```python
from build123d import *

# Parameters (mm, degrees)
F0_R     = 5.624793
F0_R_2   = 8.743876
F0_R_3   = 6.820271
F0_R_4   = 3.661746
F0_R_5   = 5.429622
F0_R_6   = 8.809277
F0_R_7   = 6.306028
F0_R_8   = 3.649185
F0_R_9   = 9.51591
F0_R_10  = 3.388182
F0_R_11  = 3.649186
F0_R_12  = 4.291104
F0_R_13  = 3.488347
F0_R_14  = 4.625832
F0_R_15  = 4.5204
F0_R_16  = 5.057367
F1_DEPTH = 7.62


with BuildPart() as f1:
    # F0 (on Top) → F1 (new body)
    with BuildSketch(Plane.XY):
        with BuildLine():
            ThreePointArc((38.1, 26.47022), (28.9765, 28.732993), (28.190642, 38.1))
            Line((28.190642, 38.1), (16.499434, 38.1))
            ThreePointArc((16.499434, 38.1), (16.874, 36.915099), (17.000607, 35.678871))
            ThreePointArc((17.000607, 35.678871), (9.665649, 29.706748), (5.304319, 38.1))
            Line((5.304319, 38.1), (-38.1, 38.1))
            Line((-38.1, 38.1), (-38.1, 17.180183))
            ThreePointArc((-38.1, 17.180183), (-32.694602, 14.941194), (-30.455614, 9.535796))
            ThreePointArc((-30.455614, 9.535796), (-32.694602, 4.130398), (-38.1, 1.89141))
            Line((-38.1, 1.89141), (-38.1, -13.310762))
            ThreePointArc((-38.1, -13.310762), (-34.005794, -13.280793), (-31.949991, -16.821569))
            ThreePointArc((-31.949991, -16.821569), (-34.005794, -20.362345), (-38.1, -20.332376))
            Line((-38.1, -20.332376), (-38.1, -26.536592))
            ThreePointArc((-38.1, -26.536592), (-28.827146, -26.010312), (-24.032091, -33.964571))
            ThreePointArc((-24.032091, -33.964571), (-24.287465, -36.092705), (-25.039087, -38.1))
            Line((-25.039087, -38.1), (-6.594518, -38.1))
            ThreePointArc((-6.594518, -38.1), (-5.905659, -25.985243), (4.486227, -32.25027))
            ThreePointArc((4.486227, -32.25027), (3.666791, -35.557694), (1.398047, -38.1))
            Line((1.398047, -38.1), (38.1, -38.1))
            Line((38.1, -38.1), (38.1, -34.461013))
            ThreePointArc((38.1, -34.461013), (22.042395, -27.750231), (38.1, -21.039449))
            Line((38.1, -21.039449), (38.1, 7.983235))
            ThreePointArc((38.1, 7.983235), (29.755205, 13.178684), (38.1, 18.374132))
            Line((38.1, 18.374132), (38.1, 26.47022))
        make_face()
        with Locations((-27.455587, -5.678618)):
            Circle(F0_R, mode=Mode.SUBTRACT)
        with Locations((-17.169787, -20.250168)):
            Circle(F0_R_2, mode=Mode.SUBTRACT)
        with Locations((-11.598311, -3.535743)):
            Circle(F0_R_3, mode=Mode.SUBTRACT)
        with Locations((10.044727, -23.035906)):
            Circle(F0_R_4, mode=Mode.SUBTRACT)
        with Locations((0, -18.321581)):
            Circle(F0_R_5, mode=Mode.SUBTRACT)
        with Locations((8.544715, -1.607155)):
            Circle(F0_R_6, mode=Mode.SUBTRACT)
        with Locations((24.401991, -10.392943)):
            Circle(F0_R_7, mode=Mode.SUBTRACT)
        with Locations((-4.312536, 6.750058)):
            Circle(F0_R_8, mode=Mode.SUBTRACT)
        with Locations((-19.526949, 19.178735)):
            Circle(F0_R_9, mode=Mode.SUBTRACT)
        with Locations((-32.812774, 31.607412)):
            Circle(F0_R_10, mode=Mode.SUBTRACT)
        with Locations((-2.598236, 26.893085)):
            Circle(F0_R_11, mode=Mode.SUBTRACT)
        with Locations((-13.741186, 33.107422)):
            Circle(F0_R_12, mode=Mode.SUBTRACT)
        with Locations((11.759028, 12.535821)):
            Circle(F0_R_13, mode=Mode.SUBTRACT)
        with Locations((24.616279, 8.464358)):
            Circle(F0_R_14, mode=Mode.SUBTRACT)
        with Locations((7.25899, 21.964472)):
            Circle(F0_R_15, mode=Mode.SUBTRACT)
        with Locations((26.544867, 23.678772)):
            Circle(F0_R_16, mode=Mode.SUBTRACT)
    extrude(amount=F1_DEPTH)


solid = f1.part
```
Design review of the part built by this model. Coordinates are the model's own, in mm. A direction names the side the tool comes from. Give positions to 0.01 mm unless a question says otherwise; leave off trailing zeros. Order: outer loops, then holes, each group sorted by start corner. A loop starts at its lowest first (then second) coordinate and runs counter-clockwise, first axis right, second up. Notation, with made-up numbers: (4.25, 38) -> (24.25, 38) arc R23 ccw to (24.25, 55) -> close; hole circle Ø4 at (43.25, 72.25). An arc over 180 degrees is marked (long way). Write item = value, one per line. Start each with the question number.
(1) We need section B-B on z = 5.75. State how many separate pieces and enclosed holes the cut face has, plus the area to 3 significant figures.
(2) We need section A-A on x = -20. Write out the cut boundary in (y, z), plus the area to 3 significant figures.
(3) For pin 1 (11.5 mm diameter, centred on x = -2.6, y = -32.25, fed in from -Z); pin 2 (1.5 mm diameter, centred on x = -2.5, z = 2.5, fed in from -Y); pin 3 (4 mm diameter, centred on y = 13, z = 6.5, fed in from -X), all flat-tipped, find the tip position at first contact; note any pin that passes through.
(4) For faces 5 (the face through (16.87, 36.93, 3.76)), 6 (the face through (-38.1, -6, 4)), list the 3-axis set-ups (+Z, -Z, +X, -X, +Y, -Y) from which the entire face can be reached by the end or side of a thin tool; tool diameter is ignored.
(5) Mouldability with a two-part tool opening along X and no side actions: class faces 1 (the face through (-38.1, 28, 4)), 2 (the face through (18.1, -10.12, 3.76)), 3 (the face through (-17, -7.7, 3.8)), 4 (the face through (-1, 1, 0)) as +X half, -X half, draft (parallel to the pull), parting line (faces both ways), or undercut.
(6) To check wall thickness, follow line 1 along Y through (x, z) = (-21.5, 6.5); line 2 along Y through (x, z) = (-31.5, 4.5); line 3 along Y through (x, z) = (-7, 4). State the ranges of each line that lie inside material, in increasing order.
Numbers:
q1.separate_pieces = 1
q1.enclosed_holes = 16
q1.area = 3,120 mm^2
q2.outline = (-38.1, 0) -> (-28.52, 0) -> (-28.52, 7.62) -> (-38.1, 7.62) -> close; (-11.98, 0) -> (9.67, 0) -> (9.67, 7.62) -> (-11.98, 7.62) -> close; (28.68, 0) -> (38.1, 0) -> (38.1, 7.62) -> (28.68, 7.62) -> close
q2.area = 310 mm^2
q3.pin_1 = through
q3.pin_2 = -25.22
q3.pin_3 = -32.75
q4.face_5 = +Z, -Z
q4.face_6 = +Z, -Z, -X, +Y, -Y
q5.face_1 = -X half
q5.face_2 = undercut
q5.face_3 = undercut
q5.face_4 = draft
q6.line_1 = -38.1 to -27.85, -12.65 to 9.87, 28.49 to 38.1
q6.line_2 = -25.1 to -9.59, -1.77 to 5.68, 13.39 to 28.48, 34.73 to 38.1
q6.line_3 = -38.1 to -37.8, -26.7 to -8.57, 1.5 to 4.28, 9.22 to 38.1
